from build123d import *

# Parameters (mm, degrees)
SKETCH1_R           = 330
BOSS_EXTRUDE1_DEPTH = 80
BOSS_EXTRUDE2_START = -80
BOSS_EXTRUDE2_DEPTH = 80
SKETCH7_W           = 110
SKETCH7_H           = 80
BOSS_EXTRUDE3_DEPTH = 650.38438807
SKETCH9_W           = 110
SKETCH9_H           = 80
CUT_EXTRUDE4_DEPTH  = 12
SKETCH10_R          = 31
CUT_EXTRUDE5_DEPTH  = 13


with BuildPart() as part:
    # Sketch1 → Boss-Extrude1 (new body)
    with BuildSketch(Plane(origin=(0, 0, 0), x_dir=(1, 0, 0), z_dir=(0, 1, 0))):
        with Locations(Location((0, 0, 0), (0, 0, 270))):
            Circle(SKETCH1_R)
    extrude(amount=BOSS_EXTRUDE1_DEPTH)

    # Sketch6 → Boss-Extrude2 (add)
    with BuildSketch(Plane(origin=(0, 80, 0), x_dir=(1, 0, 0), z_dir=(0, 1, 0)).offset(BOSS_EXTRUDE2_START)):
        with BuildLine():
            Line((-272.236110757, -194.454364826), (-275.771644663, -197.989898732))
            Line((-275.771644663, -197.989898732), (-197.989898732, -275.771644663))
            Line((-197.989898732, -275.771644663), (-194.454364826, -272.236110757))
            Line((-194.454364826, -272.236110757), (-191.190634332, -268.972380262))
            ThreePointArc((-191.190634332, -268.972380262), (-233.345237792, -233.345237792), (-268.972380262, -191.190634332))
            Line((-268.972380262, -191.190634332), (-272.236110757, -194.454364826))
        make_face()
    extrude(amount=BOSS_EXTRUDE2_DEPTH)

    # Sketch7 → Boss-Extrude3 (add)
    with BuildSketch(Plane(origin=(229.809703886, 0, -229.809703886), x_dir=(0.7071067811865476, 0, 0.7071067811865476), z_dir=(-0.7071067811865476, 0, 0.7071067811865476))):
        with Locations((0, 40)):
            Rectangle(SKETCH7_W, SKETCH7_H)
    extrude(amount=BOSS_EXTRUDE3_DEPTH)

    # Sketch9 → Cut-Extrude4 (cut)
    with BuildSketch(Plane(origin=(229.809703886, 0, -229.809703886), x_dir=(0.7071067811865476, 0, 0.7071067811865476), z_dir=(-0.7071067811865476, 0, 0.7071067811865476))):
        with Locations((0, 40)):
            Rectangle(SKETCH9_W, SKETCH9_H)
    extrude(amount=-CUT_EXTRUDE4_DEPTH, mode=Mode.SUBTRACT)

    # Sketch10 → Cut-Extrude5 (cut)
    with BuildSketch(Plane(origin=(229.809703886, 0, -229.809703886), x_dir=(-0.7071067811865475, 0, -0.7071067811865477), z_dir=(0.7071067811865477, 0, -0.7071067811865475))):
        with Locations((0, 40)):
            Circle(SKETCH10_R)
    extrude(amount=-CUT_EXTRUDE5_DEPTH, mode=Mode.SUBTRACT)


solid = part.part
Work out the finished part from the listing and answer in its coordinate system (mm). Coordinates: 2 decimals unless noted, no trailing zeros. Order: outer loops, then holes, each group sorted by start corner. A loop starts at its lowest first (then second) coordinate and runs counter-clockwise, first axis right, second up. Notation, with made-up numbers: (29.25, 78) - (65.25, 78) arc R6 ccw to (65.25, 85) - close; hole circle Ø2 at (-27, 36). An arc over 180 degrees is marked (long way). Put each result on its own line as item: value. Start each with the question number.
1) Find the intervals of material crossed by line 1 (Z direction, x = 3, y = 7); line 2 (Z direction, x = -116, y = 44); line 3 (X direction, y = 60, z = -163), in increasing order. Write a range as from..to.
2) Flat-ended cylindrical pins translate along their axes: pin 1 (5 mm diameter, centred on y = 40, z = 105.5, fed in from +X); pin 2 (1.5 mm diameter, centred on x = 32.5, y = 20, fed in from +Z); pin 3 (12 mm diameter, centred on x = -184.5, y = 71, fed in from +Z). Find the tip coordinate at first contact, or state that the pin passes through.
3) Find section C-C (z = 246). Give the vertices of the cut face in (x, y).
4) Find section D-D (y = 62). Give the vertices of the cut face in (x, z), plus the area to 3 significant figures.
5) For a pull along Y with two mould halves and no side action, classify faces 1 (the flat face through (220.924, 40.434, -220.31)), 2 (the flat face through (5, 0, -5)), 3 (the flat face through (211.98, 58.34, -247.64)) as released by +Y, released by -Y, zero draft, split by the parting line, or undercut.
6) Find section B-B (x = -135.5). Give the vertices of the cut face in (y, z).
7) Find section A-A (y = 21.5). Give the vertices of the cut face in (x, z).
Results list:
1. line 1: z = -329.99..329.99
1. line 2: z = -308.94..308.94
1. line 3: x = -286.93..286.93
2. pin 1: stops at x = 313.51
2. pin 2: stops at z = 328.47
2. pin 3: stops at z = 277.56
3. outline: (-227.76, 0) - (219.96, 0) - (219.96, 80) - (-227.76, 80) - close
4. outline: (-275.77, 197.99) - (-268.97, 191.19) arc R330 ccw to (191.19, -268.97) - (190.92, -268.7) - (214.37, -245.25) - (205.17, -236.06) - (236.06, -205.17) - (245.25, -214.37) - (268.7, -190.92) - (268.97, -191.19) arc R330 ccw to (-191.19, 268.97) - (-197.99, 275.77) - close
4. area: 342,000 mm^2
5. face 1: undercut
5. face 2: released by -Y
5. face 3: zero draft
6. outline: (0, -300.9) - (80, -300.9) - (80, 300.9) - (0, 300.9) - close
7. outline: (-275.77, 197.99) - (-268.97, 191.19) arc R330 ccw to (191.19, -268.97) - (190.92, -268.7) - (212.22, -247.4) - (203.03, -238.21) - (238.21, -203.03) - (247.4, -212.22) - (268.7, -190.92) - (268.97, -191.19) arc R330 ccw to (-191.19, 268.97) - (-197.99, 275.77) - close
